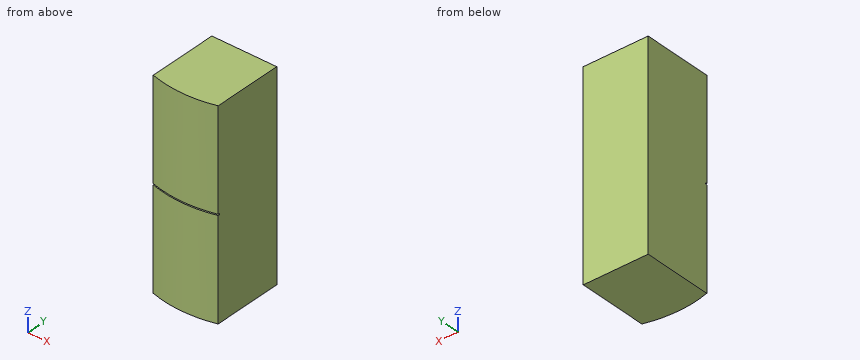
```python
from build123d import *

# Parameters (mm, degrees)
F1_DEPTH = 850
F2_W     = 550
F2_H     = 575
F3_DEPTH = 10
F4_W     = 550
F4_H     = 575
F5_DEPTH = 850


with BuildPart() as f1:
    # F0 (on Top) → F1 (new body)
    with BuildSketch(Plane.XY):
        with BuildLine():
            Line((-277.06279, 422.74684), (-277.06279, -167.25316))
            ThreePointArc((-277.06279, -167.25316), (-2.06279, -205.808933), (272.93721, -167.25316))
            Line((272.93721, -167.25316), (272.93721, 422.74684))
            Line((272.93721, 422.74684), (-277.06279, 422.74684))
        make_face()
    extrude(amount=F1_DEPTH)

    # F2 (on face) → F3 (join)
    with BuildSketch(Plane.XY.offset(850)):
        with Locations((-2.06279, 135.24684)):
            Rectangle(F2_W, F2_H)
    extrude(amount=F3_DEPTH)

    # F4 (on face) → F5 (join)
    with BuildSketch(Plane.XY.offset(860)):
        with Locations((-2.06279, 135.24684)):
            Rectangle(F4_W, F4_H)
        with BuildLine():
            Line((272.93721, -152.25316), (-277.06279, -152.25316))
            Line((-277.06279, -152.25316), (-277.06279, -167.25316))
            ThreePointArc((-277.06279, -167.25316), (-2.06279, -205.808933), (272.93721, -167.25316))
            Line((272.93721, -167.25316), (272.93721, -152.25316))
        make_face()
    extrude(amount=F5_DEPTH)


solid = f1.part
```
Read the model definition and answer for the solid it produces. Units are mm, in the model's axes. Give positions to 0.01 mm unless a question says otherwise; leave off trailing zeros. Loops run counter-clockwise (first coordinate to the right, second up) from the corner with the lowest first, then second, coordinate; pieces in that order, holes last.
Item 1: Find the intervals of material crossed by line 1 along Y through (x, z) = (-7.5, 1377.5); line 2 along Y through (x, z) = (-164, 227.5), in increasing order.
Item 2: The part is cut by section B-B (z = 1336.5). Write down the section's boundary in (x, y), and give its area (3 significant figures).
Item 3: The part is cut by section A-A (x = -229.5). Write down the section's boundary in (y, z).
Item 4: Each of these flat-tipped pins is pushed along its axis until it touches: pin 1 Ø5 at (x, y) = (196, 206) entering from -Z; pin 2 Ø5 at (x, z) = (-113, 855) entering from -Y. Where does it stop, or does it pass through?
Item 5: The part is cut by section C-C (x = 214). Write down the section's boundary in (y, z), and give its area (3 significant figures).
Taken from the geometry:
1. line 1: y = -205.79 to 422.75
1. line 2: y = -192.61 to 422.75
2. outline: (-277.06, -167.25) arc R1000 ccw to (272.94, -167.25) - (272.94, 422.75) - (-277.06, 422.75) - close
2. area: 339,000 mm2
3. outline: (-179.6, 0) - (422.75, 0) - (422.75, 1710) - (-179.6, 1710) - (-179.6, 860) - (-152.25, 860) - (-152.25, 850) - (-179.6, 850) - close
4. pin 1: stops at z = 0
4. pin 2: stops at y = -152.25
5. outline: (-182.19, 0) - (422.75, 0) - (422.75, 1710) - (-182.19, 1710) - (-182.19, 860) - (-152.25, 860) - (-152.25, 850) - (-182.19, 850) - close
5. area: 1,030,000 mm2
